```python
from build123d import *

# Parameters (mm, degrees)
F0_W     = 6.1
F0_H     = 4.65
F1_DEPTH = 2.195
F3_W     = 0.2
F3_H     = 0.2
F4_DEPTH = 10


# Not quite as in the source:
# - a feature of the source that left no trace in its solid (it failed there, or was rolled back) is left out


with BuildPart() as f1:
    # F0 (on Front) → F1 (new body, symmetric)
    with BuildSketch(Plane.XZ):
        Rectangle(F0_W, F0_H)
    extrude(amount=F1_DEPTH, both=True)

    # F3 (on face) → F4 (join)
    with BuildSketch(Plane.XY.offset(2.325)):
        with Locations((0.8, 1.055)):
            Rectangle(F3_W, F3_H)
        with Locations((-0.8, 1.055)):
            Rectangle(F3_W, F3_H)
        with Locations((0.8, -1.055)):
            Rectangle(F3_W, F3_H)
        with Locations((-0.8, -1.055)):
            Rectangle(F3_W, F3_H)
    extrude(amount=F4_DEPTH)


solid = f1.part
```
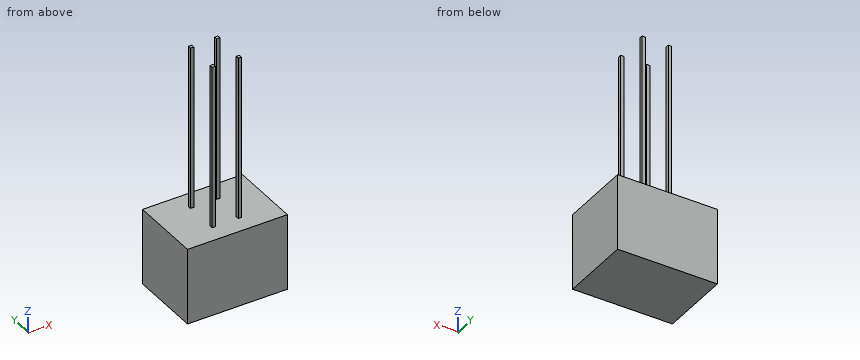
Read the model definition and answer for the solid it produces. Units are mm, in the model's axes. Round coordinates to 2 decimals unless told otherwise and drop trailing zeros. Write each loop counter-clockwise with the first axis right and the second up, starting at its lowest first coordinate (ties: lowest second). Pieces come first, ordered by that corner, then holes. Notation, with made-up numbers: (-3, 51.5) - (3, 51.5) arc R15 ccw to (3, 60.5) - close; hole circle Ø10 at (67.25, 42). An arc over 180 degrees is marked (long way). One line per item, written item: value.
Q1. Find section C-C (y = 1.8). Determine the outline of the cut face in (x, z) (3 decimals), and give its area (3 significant figures).
The answers:
outline: (-3.05, -2.325) - (3.05, -2.325) - (3.05, 2.325) - (-3.05, 2.325) - close
area: 28.4 mm2
Q2. Straight lines are drawn through the part: line 1 (Y direction, x = -0.75, z = 11.75) (3 decimals); line 2 (Z direction, x = 0, y = -1.6) (3 decimals). For each, find the intervals that lie inside material, in ascending order. Write a range as from..to.
The answers:
line 1: y = -1.155..-0.955, 0.955..1.155
line 2: z = -2.325..2.325
Q3. Each of these flat-tipped pins is pushed along its axis until it touches: P1, Ø1, axis at y = -0.5, z = 8, coming from the +X side; P2, Ø1, axis at x = -2, y = -1.5, coming from the +Z side (3 decimals); P3, Ø3, axis at x = 0, z = 5.5, coming from the -Y side (3 decimals); P4, Ø1.3, axis at x = 0.5, y = -1, coming from the +Z side (3 decimals). Where does it stop, or does it pass through?
The answers:
P1: stops at x = 0.9
P2: stops at z = 2.325
P3: stops at y = -1.155
P4: stops at z = 12.325
Q4. Find section B-B (x = 0.5). Determine the outline of the cut face in (y, z) (3 decimals), and give its area (3 significant figures).
The answers:
outline: (-2.195, -2.325) - (2.195, -2.325) - (2.195, 2.325) - (-2.195, 2.325) - close
area: 20.4 mm2
Q5. Find section A-A (z = 3.75). Determine the outline of the cut face in (x, y) (3 decimals), and give its area (3 significant figures).
The answers:
outline: (-0.9, -1.155) - (-0.7, -1.155) - (-0.7, -0.955) - (-0.9, -0.955) - close; (-0.9, 0.955) - (-0.7, 0.955) - (-0.7, 1.155) - (-0.9, 1.155) - close; (0.7, -1.155) - (0.9, -1.155) - (0.9, -0.955) - (0.7, -0.955) - close; (0.7, 0.955) - (0.9, 0.955) - (0.9, 1.155) - (0.7, 1.155) - close
area: 0.160 mm2
